from build123d import *

# Parameters (mm, degrees)
F0_R     = 12.7
F0_R_2   = 10.16
F1_DEPTH = 6.35
F2_R     = 17.5976362049
F2_R_2   = 12.7
F3_DEPTH = 5.08
F5_DEPTH = 6.35
F7_DEPTH = 6.35


with BuildPart() as f1:
    # F0 (on Top) → F1 (new body, symmetric)
    with BuildSketch(Plane.XY):
        Polygon((17.5976362049, 0), (8.7988181024, 15.24), (-8.7988181024, 15.24), (-17.5976362049, 0), (-8.7988181024, -15.24), (8.7988181024, -15.24), align=None)
        Circle(F0_R, mode=Mode.SUBTRACT)
        Circle(F0_R)
        Circle(F0_R_2, mode=Mode.SUBTRACT)
    extrude(amount=F1_DEPTH, both=True)

    # F2 (on Top) → F3 (cut, symmetric)
    with BuildSketch(Plane.XY):
        Circle(F2_R)
        Circle(F2_R_2, mode=Mode.SUBTRACT)
    extrude(amount=F3_DEPTH, both=True, mode=Mode.SUBTRACT)

    # F4 (on face) → F5 (cut)
    with BuildSketch(Plane.XY.offset(6.35)):
        with BuildLine():
            Line((-8.2631840954, 5.911462476), (-15.7600253185, 3.1828354198))
            Line((-15.7600253185, 3.1828354198), (-16.7479099485, 1.4717690485))
            Line((-16.7479099485, 1.4717690485), (-9.2510687255, 4.2003961048))
            ThreePointArc((-9.2510687255, 4.2003961048), (-8.7988181024, 5.08), (-8.2631840954, 5.911462476))
        make_face()
        with BuildLine():
            ThreePointArc((0.9878846301, -10.1118585808), (0, -10.16), (-0.9878846301, -10.1118585808))
            Line((-0.9878846301, -10.1118585808), (5.1235963296, -15.24))
            Line((5.1235963296, -15.24), (7.0993655897, -15.24))
            Line((7.0993655897, -15.24), (0.9878846301, -10.1118585808))
        make_face()
        with BuildLine():
            Line((9.6485443588, 13.7682309515), (8.2631840954, 5.911462476))
            ThreePointArc((8.2631840954, 5.911462476), (8.7988181024, 5.08), (9.2510687255, 4.2003961048))
            Line((9.2510687255, 4.2003961048), (10.6364289889, 12.0571645802))
            Line((10.6364289889, 12.0571645802), (9.6485443588, 13.7682309515))
        make_face()
    extrude(amount=-F5_DEPTH, mode=Mode.SUBTRACT)

    # F6 (on face) → F7 (cut)
    with BuildSketch(Plane(origin=(0, 0, -6.35), x_dir=(1, 0, 0), z_dir=(0, 0, -1))):
        with BuildLine():
            Line((9.6485443588, 13.7682309515), (8.2631840954, 5.911462476))
            ThreePointArc((8.2631840954, 5.911462476), (8.7988181024, 5.08), (9.2510687255, 4.2003961048))
            Line((9.2510687255, 4.2003961048), (10.6364289889, 12.0571645802))
            Line((10.6364289889, 12.0571645802), (9.6485443588, 13.7682309515))
        make_face()
        with BuildLine():
            Line((-8.2631840954, 5.911462476), (-15.7600253185, 3.1828354198))
            Line((-15.7600253185, 3.1828354198), (-16.7479099485, 1.4717690485))
            Line((-16.7479099485, 1.4717690485), (-9.2510687255, 4.2003961048))
            ThreePointArc((-9.2510687255, 4.2003961048), (-8.7988181024, 5.08), (-8.2631840954, 5.911462476))
        make_face()
        with BuildLine():
            ThreePointArc((0.9878846301, -10.1118585808), (0, -10.16), (-0.9878846301, -10.1118585808))
            Line((-0.9878846301, -10.1118585808), (5.1235963296, -15.24))
            Line((5.1235963296, -15.24), (7.0993655897, -15.24))
            Line((7.0993655897, -15.24), (0.9878846301, -10.1118585808))
        make_face()
    extrude(amount=-F7_DEPTH, mode=Mode.SUBTRACT)


solid = f1.part
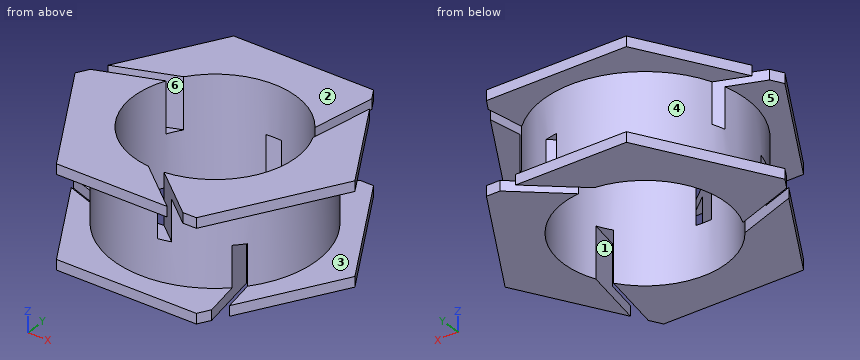
Here's how the part is built. I have some questions about the finished solid (model axes, mm). Face numbers are marked on the shaded views. A direction names the side the tool comes from. Give positions to 0.01 mm unless a question says otherwise; leave off trailing zeros. Write each loop counter-clockwise with the first axis right and the second up, starting at its lowest first coordinate (ties: lowest second). Pieces come first, ordered by that corner, then holes. Notation, with made-up numbers: (-4.75, -37.75) -> (8.25, -37.75) arc R18 ccw to (8.25, -12.75) -> close; hole circle Ø4 at (-19.5, 79). An arc over 180 degrees is marked (long way). Use one line per item in the form item = value. Start each with the question number.
1. Imagine slicing it at A-A on y = -5. List the corners of the cut face in (x, z) for me.
2. If I drill on L1, parallel to Z at x = -15, y = 1; L2, parallel to X at y = 0, z = 1.75; L3, parallel to Y at x = 11, z = -3, over which ranges is the centre line in solid material (lowest first)?
3. Imagine slicing it at B-B on x = 0. List the corners of the cut face in (y, z) for me, plus the area to 3 significant figures.
4. Thinking about a two-plate mould opening in Y: for the marked faces 4, 5 and 6, which applies, +Y half, -Y half, draft (parallel to the pull), parting line (faces both ways), or undercut?
5. On a 3-axis mill with a long thin cutter (end or side, diameter ignored), from which of +Z, -Z, +X, -X, +Y, -Y can I reach the whole of each face in a straight line? I mean the marked faces 1, 2 and 3. Say none if no direction works.
6. Imagine slicing it at C-C on z = 2.5. List the corners of the cut face in (x, y) for me, plus the area to 3 significant figures.
7. Will these pins go through, and if not, where does the flat tip stop? pin 1 Ø3 at (y, z) = (10, -2) entering from -X; pin 2 Ø4 at (y, z) = (-2, -4.5) entering from -X; pin 3 Ø0.8 at (x, y) = (9, 6.5) entering from +Z.
8. Imagine slicing it at D-D on y = -1. List the corners of the cut face in (x, z) for me, plus the area to 3 significant figures.
Entries:
q1.outline = (-14.71, -6.35) -> (-10.77, -6.35) -> (-10.77, 0) -> (-8.84, 0) -> (-8.84, 6.35) -> (-14.71, 6.35) -> (-14.71, 5.08) -> (-11.67, 5.08) -> (-11.67, -5.08) -> (-14.71, -5.08) -> close; (8.84, 0) -> (9.39, 0) -> (9.39, -6.35) -> (14.71, -6.35) -> (14.71, -5.08) -> (11.67, -5.08) -> (11.67, 5.08) -> (14.71, 5.08) -> (14.71, 6.35) -> (8.84, 6.35) -> close
q2.L1 = -6.35 to -5.08, 5.08 to 6.35
q2.L2 = -12.7 to -10.16, 10.16 to 12.7
q2.L3 = -6.35 to 6.35
q3.outline = (-15.24, -6.35) -> (-10.16, -6.35) -> (-10.16, 0) -> (-10.94, 0) -> (-10.94, 6.35) -> (-15.24, 6.35) -> (-15.24, 5.08) -> (-12.7, 5.08) -> (-12.7, -5.08) -> (-15.24, -5.08) -> close; (10.16, 0) -> (10.94, 0) -> (10.94, -6.35) -> (15.24, -6.35) -> (15.24, -5.08) -> (12.7, -5.08) -> (12.7, 5.08) -> (15.24, 5.08) -> (15.24, 6.35) -> (10.16, 6.35) -> close
q3.area = 67.5 mm²
q4.face_4 = parting line
q4.face_5 = draft
q4.face_6 = undercut
q5.face_1 = -Z
q5.face_2 = +Z, +X, -X, +Y, -Y
q5.face_3 = +X
q6.outline = (-12.32, 3.08) arc R12.7 ccw to (1.92, -12.55) -> (-0.99, -10.11) arc R10.16 cw to (-9.25, 4.2) -> close; (-11.83, 4.61) -> (-8.26, 5.91) arc R10.16 cw to (8.26, 5.91) -> (8.83, 9.13) arc R12.7 ccw to start; (0.99, -10.11) -> (3.49, -12.21) arc R12.7 ccw to (9.91, 7.94) -> (9.25, 4.2) arc R10.16 cw to start
q6.area = 169 mm²
q7.pin_1 = -9.44
q7.pin_2 = -17.55
q7.pin_3 = 0
q8.outline = (-17.02, -6.35) -> (-10.11, -6.35) -> (-10.11, 6.35) -> (-17.02, 6.35) -> (-17.02, 5.08) -> (-12.66, 5.08) -> (-12.66, -5.08) -> (-17.02, -5.08) -> close; (10.11, -6.35) -> (17.02, -6.35) -> (17.02, -5.08) -> (12.66, -5.08) -> (12.66, 5.08) -> (17.02, 5.08) -> (17.02, 6.35) -> (10.11, 6.35) -> close
q8.area = 86.9 mm²
